from build123d import *

# Parameters (mm, degrees)
SKETCH_W     = 51
SKETCH_H     = 10
PAD_DEPTH    = 1.5
SKETCH001_W  = 22
SKETCH001_H  = 7.32541
POCKET_DEPTH = 5
SKETCH002_W  = 51
SKETCH002_H  = 6
PAD001_DEPTH = 2


with BuildPart() as part:
    # Sketch → Pad (new body)
    with BuildSketch(Plane.XZ):
        with Locations((25.5, 5)):
            Rectangle(SKETCH_W, SKETCH_H)
    extrude(amount=PAD_DEPTH)

    # Sketch001 (on Face6 of Pad) → Pocket (cut)
    with BuildSketch(Plane.XZ.offset(1.5)):
        with Locations((25.5, 3.662705)):
            Rectangle(SKETCH001_W, SKETCH001_H)
    extrude(amount=-POCKET_DEPTH, mode=Mode.SUBTRACT)

    # Sketch002 (on Face6 of Pocket) → Pad001 (join)
    with BuildSketch(Plane(origin=(0, 0, 10), x_dir=(-1, 0, 0), z_dir=(0, 0, 1))):
        with Locations((-25.5, 0.75)):
            Rectangle(SKETCH002_W, SKETCH002_H)
    extrude(amount=PAD001_DEPTH)


solid = part.part
Input: part model. Units: mm. Frame: model coordinates. A direction names the side the tool comes from. Coordinates: 2 decimals unless noted, no trailing zeros. Loops run counter-clockwise (first coordinate to the right, second up) from the corner with the lowest first, then second, coordinate; pieces in that order, holes last. Notation, with made-up numbers: (56.25, 59) -> (114.25, 59) arc R19 ccw to (114.25, 68) -> close; hole circle Ø7 at (63, 56.5). An arc over 180 degrees is marked (long way). Write item = value, one per line. Start each with the question number.
Item 1: Cut plane B-B, the plane x = 18. Return loops of the section in (y, z).
Item 2: Cut plane A-A, the plane z = 3. Return loops of the section in (x, y).
Item 3: Cut plane D-D, the plane x = 45. Return loops of the section in (y, z).
Item 4: First-contact query: P1, Ø5, axis at x = 34.5, z = 5, coming from the -Y side; P2, Ø2.5, axis at x = 16, y = 1.5, coming from the -Z side; P3, Ø3, axis at x = 22.5, z = 7, coming from the +Y side. Flat tips, straight axial feed; report the tip coordinate or a pass-through.
Item 5: Mould query, pull axis X, two halves, no side actions, for faces 5 (the face through (26, -1, 12)), 6 (the face through (36.5, -1, 4)), 7 (the face through (0, -1, 7)). Classes: pulls with the +X half, pulls with the -X half, needs draft (parallel to the pull), parting line crosses it, or undercut.
Item 6: Material intervals for line 1 (X direction, y = -1.05, z = 1.75); line 2 (Z direction, x = 35, y = -2.1); line 3 (Y direction, x = 38.5, z = 8.25), sorted ascending.
Item 7: Reachability of faces 1 (the face through (25, 0, 8)), 2 (the face through (26, -3, 10)), 3 (the face through (7, -1, 0)), 4 (the face through (14.5, -1, 4)) from +Z, -Z, +X, -X, +Y, -Y: full face, straight path, thin tool, end or side. Return the list, or none.
Item 8: Cut plane C-C, the plane y = -2.95. Return loops of the section in (x, z).
Ans:
q1.outline = (-3.75, 10) -> (-1.5, 10) -> (-1.5, 7.33) -> (0, 7.33) -> (0, 10) -> (2.25, 10) -> (2.25, 12) -> (-3.75, 12) -> close
q2.outline = (0, -1.5) -> (14.5, -1.5) -> (14.5, 0) -> (0, 0) -> close; (36.5, -1.5) -> (51, -1.5) -> (51, 0) -> (36.5, 0) -> close
q3.outline = (-3.75, 10) -> (-1.5, 10) -> (-1.5, 0) -> (0, 0) -> (0, 10) -> (2.25, 10) -> (2.25, 12) -> (-3.75, 12) -> close
q4.P1 = -1.5
q4.P2 = 10
q4.P3 = 0
q5.face_5 = needs draft
q5.face_6 = undercut
q5.face_7 = pulls with the -X half
q6.line_1 = 0 to 14.5, 36.5 to 51
q6.line_2 = 10 to 12
q6.line_3 = -1.5 to 0
q7.face_1 = -Z, +X, -X, +Y
q7.face_2 = -Z, +X, -X, -Y
q7.face_3 = -Z, +X, -X, +Y, -Y
q7.face_4 = -Z, +Y, -Y
q8.outline = (0, 10) -> (51, 10) -> (51, 12) -> (0, 12) -> close
